Can you work these out from the model? Positions are in its coordinate system, mm. A direction names the side the tool comes from. Coordinates: 2 decimals unless noted, no trailing zeros. Loops run counter-clockwise (first coordinate to the right, second up) from the corner with the lowest first, then second, coordinate; pieces in that order, holes last. Notation, with made-up numbers: (-8, 8) -> (0, 8) arc R23 cw to (0, 38) -> close; hole circle Ø5 at (-21.75, 1). An arc over 180 degrees is marked (long way). Use one line per item in the form item = value. Start each with the question number.
(1) Thinking about a two-plate mould opening in X: for faces 4 (the flat face through (431.844, 445, -226)), 5 (the flat face through (13, 431.8, -231)), 6 (the flat face through (457.244, 278, -433)), which applies, released by +X, released by -X, zero draft, split by the parting line, or undercut?
(2) Imagine slicing it at A-A (z = -54). List the corners of the cut face in (x, y) for me.
(3) I need wall thicknesses on line 1 (Z direction, x = 138, y = 433); line 2 (X direction, y = 434, z = -399); line 3 (Y direction, x = 432, z = -378). Which ranges of each line are inside material? Lowest first, please. Write a range as [from, to].
(4) Imagine slicing it at B-B (x = 325.5). List the corners of the cut face in (y, z) for me, plus the area to 3 significant figures.
(5) I'm going to push flat-ended pins straight in: pin 1 (7.5 mm diameter, centred on x = 15, y = 164, fed in from -Z); pin 2 (7.5 mm diameter, centred on x = 291.5, z = -448.5, fed in from -Y); pin 3 (7.5 mm diameter, centred on x = 222.5, y = 443, fed in from +Z). Where does each tip first touch, or does it pass through?
(6) On a 3-axis mill with a long thin cutter (end or side, diameter ignored), from which of +Z, -Z, +X, -X, +Y, -Y can I reach the whole of each face in a straight line? I mean faces 1 (the flat face through (13, 226, -25.4)), 2 (the flat face through (25.4, 226, -13)), 3 (the flat face through (25.4, 445, -231)). Say none if no direction works.
Autodesk Inventor part; units mm, degrees
ref_plane "YZ Plane" through (0, 0, 0) normal (1, 0, 0) x (0, 1, 0)
ref_plane "XZ Plane" through (0, 0, 0) normal (0, 1, 0) x (-1, 0, 0)
ref_plane "XY Plane" through (0, 0, 0) normal (0, 0, 1) x (1, 0, 0)
sketch "Sketch1" plane through (0, 0, 0) normal (0, 1, 0) x (-1, 0, 0)
  line L0 (0, 0) -> (-457.2, 0)
  line L1 (-457.2, 0) -> (-457.2, -25.4)
  line L2 (-457.2, -25.4) -> (0, -25.4)
  line L3 (0, -25.4) -> (0, 0)
  line L4 (0, 0) -> (-25.4, 0)
  line L5 (-25.4, 0) -> (-25.4, -457.2)
  line L6 (-25.4, -457.2) -> (0, -457.2)
  line L7 (0, -457.2) -> (0, 0)
  line L8 (0, -457.2) -> (-457.2, -457.2)
  line L9 (-457.2, -457.2) -> (-457.2, -431.8)
  line L10 (-457.2, -431.8) -> (0, -431.8)
  line L11 (0, -431.8) -> (0, -457.2)
  line L12 (-457.2, 0) -> (-431.8, 0)
  line L13 (-431.8, 0) -> (-431.8, -457.2)
  line L14 (-431.8, -457.2) -> (-457.2, -457.2)
  line L15 (-457.2, -457.2) -> (-457.2, 0)
  dimension "d0" = 457.2
  dimension "d1" = 25.4
  dimension "d2" = 25.4
  dimension "d3" = 457.2
  dimension "d4" = 457.2
  dimension "d5" = 25.4
  dimension "d6" = 25.4
sketch "Sketch2" plane through (0, 0, 0) normal (0, 1, 0) x (-1, 0, 0)
  line L0 (0, 0) -> (-25.4, 0)
  line L1 (-25.4, 0) -> (-25.4, -25.4)
  line L2 (-25.4, -25.4) -> (0, -25.4)
  line L3 (0, -25.4) -> (0, 0)
  line L4 (0, -457.1579) -> (-25.4, -457.1579)
  line L5 (-25.4, -457.1579) -> (-25.4, -431.7579)
  line L6 (-25.4, -431.7579) -> (0, -431.7579)
  line L7 (0, -431.7579) -> (0, -457.1579)
  line L8 (-457.244, -457.1579) -> (-431.844, -457.1579)
  line L9 (-431.844, -457.1579) -> (-431.844, -431.7579)
  line L10 (-431.844, -431.7579) -> (-457.244, -431.7579)
  line L11 (-457.244, -431.7579) -> (-457.244, -457.1579)
  line L12 (-457.244, 0) -> (-431.844, 0)
  line L13 (-431.844, 0) -> (-431.844, -25.4)
  line L14 (-431.844, -25.4) -> (-457.244, -25.4)
  line L15 (-457.244, -25.4) -> (-457.244, 0)
  dimension "d7" = 25.4
  dimension "d8" = 25.4
  dimension "d9" = 25.4
  dimension "d10" = 25.4
  dimension "d11" = 25.4
  dimension "d12" = 25.4
  dimension "d13" = 25.4
  dimension "d14" = 25.4
sketch "Sketch3" plane through (0, 0, 0) normal (0, 0, 1) x (1, 0, 0)
  point P0 (0, 0)
sketch "Sketch4" plane through (0, 0, 0) normal (0, 0, 1) x (1, 0, 0)
  point P0 (0, 0)
extrude "Extrusion1" add sketch "Sketch1" along normal blind 25.4 contours L3 L2 L5 L0 | L5 L2 L13 L0 | L7 L10 L5 L2 | L13 L2 L1 L0 | L7 L6 L5 L10 | L13 L10 L15 L2 | L5 L8 L13 L10 | L13 L8 L9 L10
extrude "Extrusion2" add sketch "Sketch2" along normal blind 457.2
sketch "Sketch5" plane through (0, 457.2, 0) normal (0, 1, 0) x (1, 0, 0)
  line L0 (0, 0) -> (25.4, 0)
  line L1 (25.4, 0) -> (25.4, 25.4)
  line L2 (25.4, 25.4) -> (0, 25.4)
  line L3 (0, 25.4) -> (0, 0)
  line L4 (0, 457.1579) -> (25.4, 457.1579)
  line L5 (25.4, 457.1579) -> (25.4, -0.0421)
  line L6 (25.4, -0.0421) -> (0, -0.0421)
  line L7 (0, -0.0421) -> (0, 457.1579)
  line L8 (457.244, 25.4) -> (431.844, 25.4)
  line L9 (0, 0) -> (457.2, 0)
  line L10 (457.2, 0) -> (457.2, 25.4)
  line L11 (457.2, 25.4) -> (0, 25.4)
  line L12 (0, 25.4) -> (0, 0)
  line L13 (431.844, 431.7579) -> (457.244, 431.7579)
  line L14 (0, 457.1579) -> (457.2, 457.1579)
  line L15 (457.2, 457.1579) -> (457.2, 431.7579)
  line L16 (457.2, 431.7579) -> (0, 431.7579)
  line L17 (0, 431.7579) -> (0, 457.1579)
  line L18 (457.244, 0) -> (431.844, 0)
  line L19 (431.844, 0) -> (431.844, 457.2)
  line L20 (431.844, 457.2) -> (457.244, 457.2)
  line L21 (457.244, 457.2) -> (457.244, 0)
  dimension "d19" = 25.4
  dimension "d20" = 457.2
  dimension "d21" = 457.2
  dimension "d22" = 457.2
  dimension "d23" = 25.4
  dimension "d24" = 457.2
extrude "Extrusion3" add sketch "Sketch5" against normal blind 25.4 contours L3 L2 L1 L0 | L0 L5 L6 L7 | L1 L11 L19 L9 | L7 L16 L5 L2 | L19 L8 L10 L9 | L7 L4 L5 L16 | L5 L14 L19 L16 | L19 L13 L21 L8 | L10 L8 L21 L18 | L19 L14 L15 L13 | L19 L20 L21 L13 L15 L14
properties part number "Basic Frame"
Worked out:
q1.face_4 = undercut
q1.face_5 = zero draft
q1.face_6 = released by +X
q2.outline = (0, 0) -> (25.4, 0) -> (25.4, 25.4) -> (0, 25.4) -> close; (0, 431.8) -> (25.4, 431.8) -> (25.4, 457.2) -> (0, 457.2) -> close; (431.8, 0) -> (457.2, 0) -> (457.2, 25.4) -> (431.8, 25.4) -> close; (431.84, 431.8) -> (457.24, 431.8) -> (457.24, 457.2) -> (431.84, 457.2) -> close
q3.line_1 = [-457.16, -431.76], [-25.4, 0]
q3.line_2 = [0, 25.4], [431.84, 457.24]
q3.line_3 = [0, 25.4], [431.8, 457.2]
q4.outline = (0, -457.2) -> (25.4, -457.2) -> (25.4, -431.8) -> (0, -431.8) -> close; (0, -25.4) -> (25.4, -25.4) -> (25.4, 0) -> (0, 0) -> close; (431.8, -457.16) -> (457.2, -457.16) -> (457.2, -431.76) -> (431.8, -431.76) -> close; (431.8, -25.4) -> (457.2, -25.4) -> (457.2, 0) -> (431.8, 0) -> close
q4.area = 2,580 mm2
q5.pin_1 = -457.16
q5.pin_2 = 0
q5.pin_3 = 0
q6.face_1 = +X, -X
q6.face_2 = +Z, -Z
q6.face_3 = +Y, -Y
